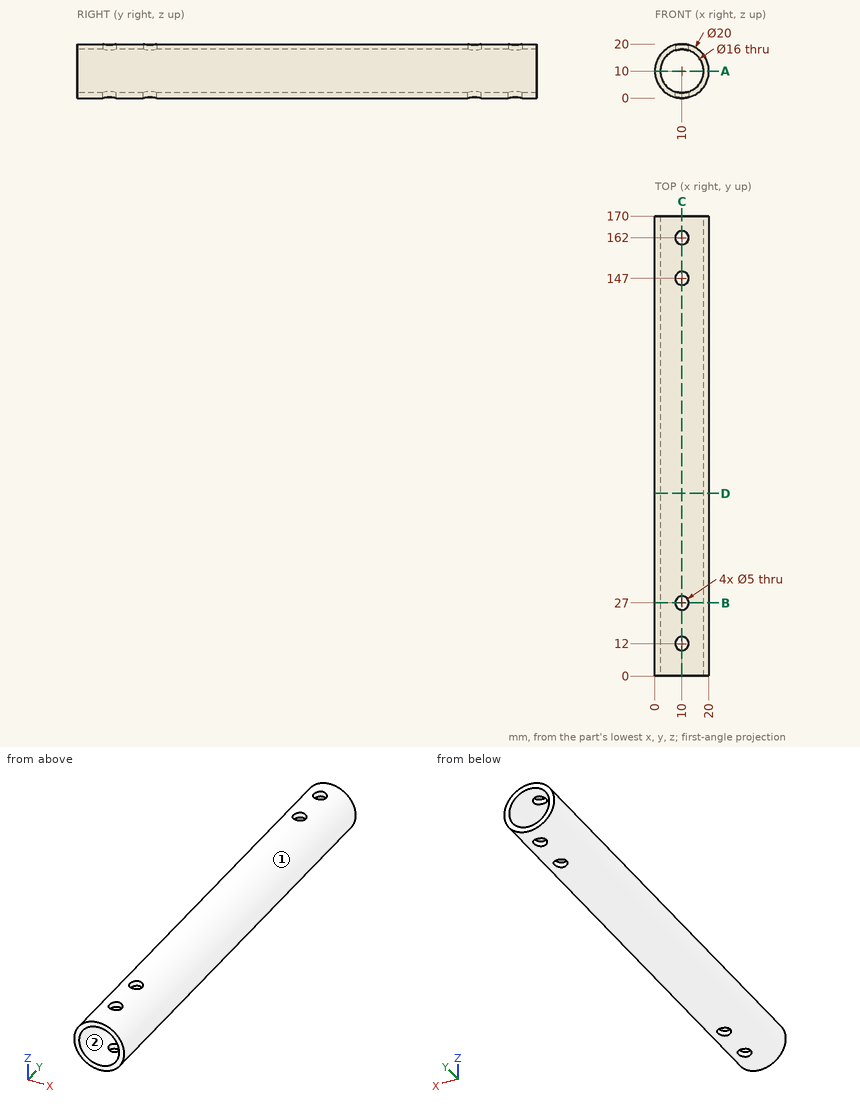
Design review of the part shown in the three views and the two pictorial views. Dimensions are in mm from the part's minimum x, y and z. Round coordinates to 2 decimals unless told otherwise and drop trailing zeros. Loops run counter-clockwise (first coordinate to the right, second up) from the corner with the lowest first, then second, coordinate; pieces in that order, holes last. Notation, with made-up numbers: (5, 52) -> (64, 52) arc R19 ccw to (64, 65) -> close; hole circle Ø7 at (-18.75, 78.25). An arc over 180 degrees is marked (long way). Use one line per item in the form item = value. Start each with the question number.
Q1. For pin 1 Ø2 at (x, y) = (7.5, 27.5) entering from +Z; pin 2 Ø1 at (y, z) = (98.5, 12.5) entering from -X; pin 3 Ø4 at (y, z) = (101.5, 7.5) entering from +X, all flat-tipped, find the tip position at first contact; note any pin that passes through.
Q2. Wall thickness on line 1 along Y through (x, z) = (10, 18.55); line 2 along Z through (x, y) = (10.5, 82); line 3 along Z through (x, y) = (4, 125.5): over which ranges is each line inside the solid? List them lowest first. Write a range as [from, to].
Q3. We need section C-C on x = 10. State how many separate pieces and enclosed holes the cut face has, then the cut area to 3 significant figures.
Q4. We need section D-D on y = 67.5. Give the boundary of the cut face in (x, z), then the cut area to 3 significant figures.
Q5. We need section A-A on z = 10. Give the boundary of the cut face in (x, y), then the cut area to 3 significant figures.
Q6. Draft analysis for pull direction X (two halves, no side actions). For the marked faces 1 and 2, state which applies: +X half, -X half, draft (parallel to the pull), parting line (faces both ways), or undercut.
Q7. We need section B-B on y = 27. Give the boundary of the cut face in (x, z), then the cut area to 3 significant figures.
Calculated:
q1.pin_1 = 19.78
q1.pin_2 = 0.2
q1.pin_3 = 19.99
q2.line_1 = [0, 9.5], [14.5, 24.5], [29.5, 144.5], [149.5, 159.5], [164.5, 170]
q2.line_2 = [0.01, 2.02], [17.98, 19.99]
q2.line_3 = [2, 4.71], [15.29, 18]
q3.separate_pieces = 10
q3.enclosed_holes = 0
q3.area = 600 mm²
q4.outline = circle Ø20 at (10, 10); hole circle Ø16 at (10, 10)
q4.area = 113 mm²
q5.outline = (0, 0) -> (2, 0) -> (2, 170) -> (0, 170) -> close; (18, 0) -> (20, 0) -> (20, 170) -> (18, 170) -> close
q5.area = 680 mm²
q6.face_1 = parting line
q6.face_2 = undercut
q7.outline = (7.5, 0.32) -> (7.5, 2.4) arc R8 cw to (7.5, 17.6) -> (7.5, 19.68) arc R10 ccw to start; (12.5, 0.32) arc R10 ccw to (12.5, 19.68) -> (12.5, 17.6) arc R8 cw to (12.5, 2.4) -> close
q7.area = 92.8 mm²
